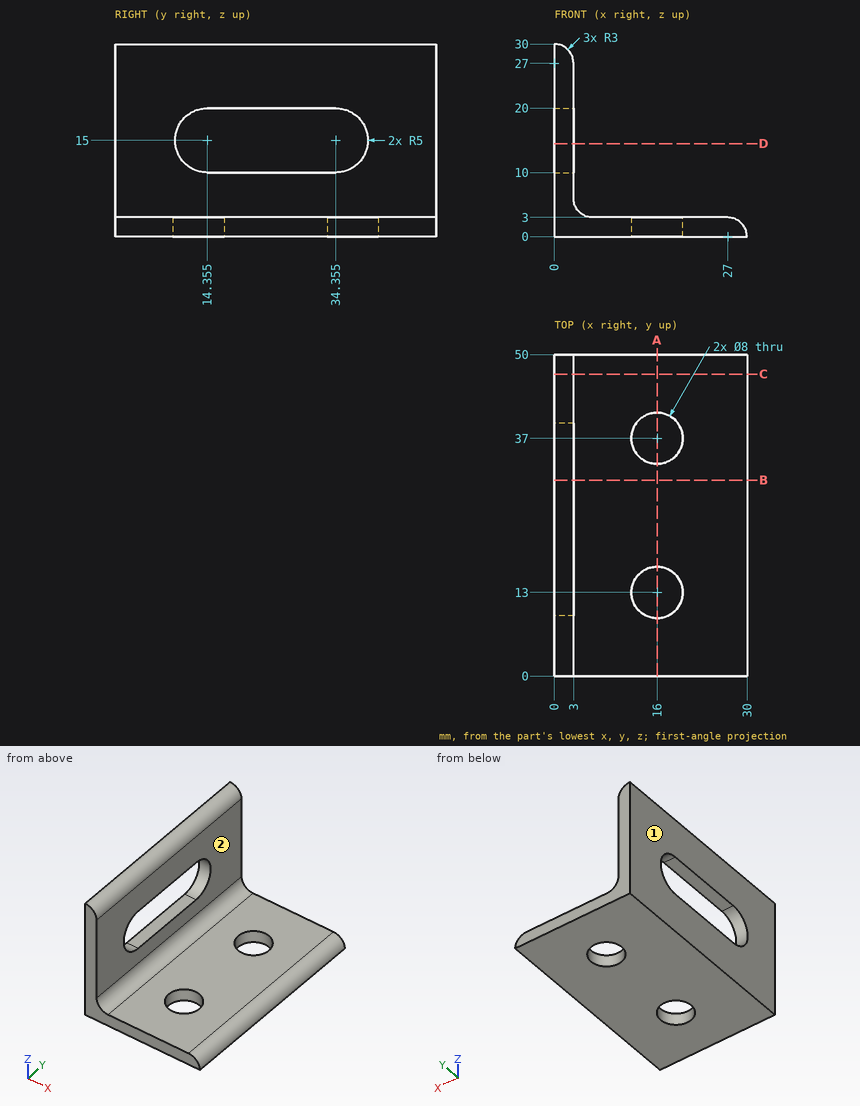
Job drawing, mm, ordinate dimensions from the low corner. One solid piece. A direction names the side the tool comes from. Coordinates: 2 decimals unless noted, no trailing zeros. Order: outer loops, then holes, each group sorted by start corner. A loop starts at its lowest first (then second) coordinate and runs counter-clockwise, first axis right, second up. Notation, with made-up numbers: (-11, 39.5) - (9, 39.5) arc R28 ccw to (9, 69.5) - close; hole circle Ø6 at (65, -19). An arc over 180 degrees is marked (long way). Write each question's results on one line, items separated by ' | '. Start each with the question number.
Item 1: Tool access for the marked faces 1 and 2: list every direction of +Z, -Z, +X, -X, +Y, -Y with a clear straight run to the whole face (end or side of a thin tool).
Item 2: Band-saw the part on B-B on y = 30.5. Write the cut outline in (x, z), and give its area (3 significant figures).
Item 3: Flat gauge pins, fed straight in: pin 1 (1.5 mm diameter, centred on x = 1, y = 27.5, fed in from +Z); pin 2 (4 mm diameter, centred on x = 3.5, z = 17.5, fed in from +Y); pin 3 (1 mm diameter, centred on x = 13.5, y = 5, fed in from +Z); pin 4 (17 mm diameter, centred on y = 37, z = 13.5, fed in from +X). Where does each tip first touch, or does it go through?
Item 4: Band-saw the part on C-C on y = 47. Write the cut outline in (x, z).
Item 5: Band-saw the part on A-A on x = 16. Write the cut outline in (y, z), and give its area (3 significant figures).
Item 6: Wall check: probe 1 along Y at (x, z) = (16, 1.45); probe 2 along Z at (x, y) = (17, 21). Give the ranges that are in metal, low to high. Write a range as [from, to].
Item 7: Band-saw the part on D-D on z = 14.5. Write the cut outline in (x, y).
Numbers:
1) face 1: +Z, -Z, -X, +Y, -Y | face 2: +Z, +X, +Y, -Y
2) outline: (0, 0) - (30, 0) arc R3 ccw to (27, 3) - (6, 3) arc R3 cw to (3, 6) - (3, 10) - (0, 10) - close; (0, 20) - (3, 20) - (3, 27) arc R3 ccw to (0, 30) - close | area: 139 mm^2
3) pin 1: z = 29.99 | pin 2: y = 50 | pin 3: z = 3 | pin 4: x = 3.17
4) outline: (0, 0) - (30, 0) arc R3 ccw to (27, 3) - (6, 3) arc R3 cw to (3, 6) - (3, 27) arc R3 ccw to (0, 30) - close
5) outline: (0, 0) - (9, 0) - (9, 3) - (0, 3) - close; (17, 0) - (33, 0) - (33, 3) - (17, 3) - close; (41, 0) - (50, 0) - (50, 3) - (41, 3) - close | area: 102 mm^2
6) probe 1: [0, 9], [17, 33], [41, 50] | probe 2: [0, 3]
7) outline: (0, 0) - (3, 0) - (3, 9.38) - (0, 9.38) - close; (0, 39.33) - (3, 39.33) - (3, 50) - (0, 50) - close
